For this review, take the finished solid that the model builds, in its own axes (mm). A direction names the side the tool comes from. Coordinates: 2 decimals unless noted, no trailing zeros. Loops run counter-clockwise (first coordinate to the right, second up) from the corner with the lowest first, then second, coordinate; pieces in that order, holes last. Notation, with made-up numbers: (62, 82.5) -> (67, 82.5) arc R25 ccw to (67, 118.5) -> close; hole circle Ø7 at (47.5, 0.5). An arc over 180 degrees is marked (long way). One line per item, written item: value.
from build123d import *

# Parameters (mm, degrees)
SKETCH1_W           = 64.77
SKETCH1_H           = 30.48
BOSS_EXTRUDE1_DEPTH = 2.54
SKETCH2_W           = 60.96
SKETCH2_H           = 53.34
BOSS_EXTRUDE2_DEPTH = 2.54
BOSS_EXTRUDE4_DEPTH = 25.4


with BuildPart() as part:
    # Sketch1 → Boss-Extrude1 (new body)
    with BuildSketch(Plane.XY):
        Rectangle(SKETCH1_W, SKETCH1_H)
    extrude(amount=BOSS_EXTRUDE1_DEPTH)



with BuildPart() as body_2:
    # Sketch2 → Boss-Extrude2 (new body)
    with BuildSketch(Plane.XZ.offset(15.24)):
        with Locations((0, -26.67)):
            Rectangle(SKETCH2_W, SKETCH2_H)
    extrude(amount=-BOSS_EXTRUDE2_DEPTH)


with BuildPart() as part_1:
    add(part.part)

    add(body_2.part)  # Boss-Extrude4 merges body 2
    # Sketch3 → Boss-Extrude4 (add)
    with BuildSketch(Plane(origin=(0, -12.7, 0), x_dir=(-1, 0, 0), z_dir=(0, -1, 0))):
        Polygon((27.94, 50.8), (27.94, 0), (30.48, 0), (30.48, 53.34), (-30.48, 53.34), (-30.48, 0), (-27.94, 0), (-27.94, 50.8), align=None)
    extrude(amount=-BOSS_EXTRUDE4_DEPTH)


solid = part_1.part
1. For faces 1 (the flat face through (-27.94, 0, -26)), 2 (the flat face through (0, -1, -53.34)), 3 (the flat face through (-30.48, -1, -26)), 4 (the flat face through (30.48, -1, -27)), 5 (the flat face through (0, 12.7, -52)), list the 3-axis set-ups (+Z, -Z, +X, -X, +Y, -Y) from which the entire face can be reached by the end or side of a thin tool; tool diameter is ignored.
Return value:
face 1: +Y
face 2: -Z, +X, -X, +Y, -Y
face 3: -Z, -X, +Y, -Y
face 4: -Z, +X, +Y, -Y
face 5: -Z, +X, -X, +Y
2. Take a section at A-A, the plane y = 11.5. Give the boundary of the cut face in (x, z) (3 decimals), and give its area (3 significant figures).
Return value:
outline: (-32.385, 0) -> (-30.48, 0) -> (-30.48, -53.34) -> (30.48, -53.34) -> (30.48, 0) -> (32.385, 0) -> (32.385, 2.54) -> (-32.385, 2.54) -> close; hole (-27.94, -50.8) -> (27.94, -50.8) -> (27.94, 0) -> (-27.94, 0) -> close
area: 577 mm2
3. Insertion check: pin 1 Ø6 at (x, z) = (-13.5, -37.5) entering from +Y; pin 2 Ø12.5 at (y, z) = (-2, -13.5) entering from -X; pin 3 Ø7.5 at (y, z) = (4.5, -19.5) entering from +X. Each pin has a flat end and moves straight along its axis. Give the tip position at first contact, or say it passes through.
Return value:
pin 1: stops at y = -12.7
pin 2: stops at x = -30.48
pin 3: stops at x = 30.48
4. The part is to be moulded in two halves that separate along X. For faces 6 (the flat face through (32.385, 0, 1)), 7 (the flat face through (0, -15.24, -26)), 8 (the flat face through (27.94, 0, -25)), 9 (the flat face through (0, 4, 0)), say which applies: pulls with the +X half, pulls with the -X half, needs draft (parallel to the pull), parting line crosses it, or undercut.
Return value:
face 6: pulls with the +X half
face 7: needs draft
face 8: undercut
face 9: undercut
5. Take a section at B-B, the plane x = 25.5. Give the boundary of the cut face in (y, z), and give its area (3 significant figures).
Return value:
outline: (-15.24, -53.34) -> (12.7, -53.34) -> (12.7, -50.8) -> (-12.7, -50.8) -> (-12.7, 0) -> (15.24, 0) -> (15.24, 2.54) -> (-15.24, 2.54) -> close
area: 277 mm2
6. Take a section at C-C, the plane z = -42. Give the boundary of the cut face in (x, y).
Return value:
outline: (-30.48, -15.24) -> (30.48, -15.24) -> (30.48, 12.7) -> (27.94, 12.7) -> (27.94, -12.7) -> (-27.94, -12.7) -> (-27.94, 12.7) -> (-30.48, 12.7) -> close
7. To check wall thickness, follow probe 1 along Z at (x, y) = (-17, 2.5); probe 2 along X at (y, z) = (6, -32); probe 3 along Y at (x, z) = (-12, -4). State the ranges of each line that lie inside material, in increasing order. Write a range as from..to.
Return value:
probe 1: z = -53.34..-50.8, 0..2.54
probe 2: x = -30.48..-27.94, 27.94..30.48
probe 3: y = -15.24..-12.7
